from build123d import *

# Parameters (mm, degrees)
SKETCH_1_R               = 9
EXTRUDE_1_DEPTH          = 7.5
SKETCH_2_R               = 5
EXTRUDE_2_DEPTH          = 6.5
SKETCH_3_R               = 3
CUT_EXTRUDE_1_DEPTH      = 19.920887928
CUT_EXTRUDE_2_DEPTH      = 19.920887928
CUT_EXTRUDE_2_DEPTH_BACK = 19.920887928
SKETCH_4_R               = 1.5
SKETCH_5_W               = 4
SKETCH_5_H               = 1
SKETCH_6_R               = 0.75
CUT_EXTRUDE_3_DEPTH      = 10
CUT_EXTRUDE_4_DEPTH      = 19.920888002
CUT_EXTRUDE_4_DEPTH_BACK = 19.920888002
SKETCH_8_W               = 6.5
SKETCH_8_H               = 0.5


with BuildPart() as part:
    # 草图1 → 凸台-拉伸1 (new body)
    with BuildSketch(Plane.XY):
        Circle(SKETCH_1_R)
    extrude(amount=EXTRUDE_1_DEPTH)

    # 草图2 → 凸台-拉伸2 (add)
    with BuildSketch(Plane.XY.offset(7.5)):
        with Locations(Location((0, 0, 0), (0, 0, 180))):
            Circle(SKETCH_2_R)
    extrude(amount=EXTRUDE_2_DEPTH)

    # 草图3 → 切除-拉伸1 (cut, through all)
    with BuildSketch(Plane.XY.offset(14)):
        Circle(SKETCH_3_R)
    extrude(amount=-CUT_EXTRUDE_1_DEPTH, mode=Mode.SUBTRACT)

    # 草图4 → 切除-拉伸2 (cut, two sides: drawn at the far end of the back side and taken through both)
    with BuildSketch(Plane(origin=(0, 0, 0), x_dir=(1, 0, 0), z_dir=(0, 1, 0)).offset(-CUT_EXTRUDE_2_DEPTH_BACK)):
        with Locations(Location((0, -11, 0), (0, 0, 270))):
            Circle(SKETCH_4_R)
    extrude(amount=CUT_EXTRUDE_2_DEPTH + CUT_EXTRUDE_2_DEPTH_BACK, mode=Mode.SUBTRACT)

    # 草图5 → 切除-旋转1 (revolve, cut)
    with BuildSketch(Plane(origin=(0, 0, 0), x_dir=(1, 0, 0), z_dir=(0, 1, 0)), mode=Mode.PRIVATE) as cut_revolve_1_sk:
        with Locations((7, -1.5)):
            Rectangle(SKETCH_5_W, SKETCH_5_H)
        with Locations((7, -6)):
            Rectangle(SKETCH_5_W, SKETCH_5_H)
    revolve(cut_revolve_1_sk.sketch.rotate(Axis((0, 0, -0.802981009), (0, 0, 1)), 180), axis=Axis((0, 0, -0.802981009), (0, 0, 1)), mode=Mode.SUBTRACT)

    # 草图6 → 切除-拉伸3 (cut)
    with BuildSketch(Plane.XY.offset(7.5)):
        with Locations((7, 0)):
            Circle(SKETCH_6_R)
    extrude(amount=-CUT_EXTRUDE_3_DEPTH, mode=Mode.SUBTRACT)

    # 草图8 → 切除-拉伸4 (cut, two sides: drawn at the far end of the back side and taken through both)
    with BuildSketch(Plane(origin=(0, 0, 0), x_dir=(0, 0, -1), z_dir=(1, 0, 0)).offset(-CUT_EXTRUDE_4_DEPTH_BACK)):
        with Locations((-10.75, 4.75)):
            Rectangle(SKETCH_8_W, SKETCH_8_H)
    extrude(amount=CUT_EXTRUDE_4_DEPTH + CUT_EXTRUDE_4_DEPTH_BACK, mode=Mode.SUBTRACT)


solid = part.part
Model file for the job. Use its own axes, mm. A direction names the side the tool comes from. Give positions to 0.01 mm unless a question says otherwise; leave off trailing zeros. Write each loop counter-clockwise with the first axis right and the second up, starting at its lowest first coordinate (ties: lowest second). Pieces come first, ordered by that corner, then holes. Notation, with made-up numbers: (35.5, -13.75) -> (69.5, -13.75) arc R32 cw to (69.5, 21.25) -> close; hole circle Ø3 at (-9, 75.5). An arc over 180 degrees is marked (long way). Write item = value, one per line.
(1) Slice it at B-B, the plane x = 7. Give the cut face in (y, z), then the cut area to 3 significant figures.
Determined:
outline = (-5.66, 0) -> (-0.75, 0) -> (-0.75, 1) -> (-5.66, 1) -> close; (-5.66, 2) -> (-0.75, 2) -> (-0.75, 5.5) -> (-5.66, 5.5) -> close; (-5.66, 6.5) -> (-0.75, 6.5) -> (-0.75, 7.5) -> (-5.66, 7.5) -> close; (0.75, 0) -> (5.66, 0) -> (5.66, 1) -> (0.75, 1) -> close; (0.75, 2) -> (5.66, 2) -> (5.66, 5.5) -> (0.75, 5.5) -> close; (0.75, 6.5) -> (5.66, 6.5) -> (5.66, 7.5) -> (0.75, 7.5) -> close
area = 54.0 mm2
(2) Mould opens along X. For faces 4 (the face through (-1.172, 8.923, 3.726)), 5 (the face through (4, 4, 2)), 6 (the face through (2.77, -1.15, 7.1)) say: released by +X, released by -X, zero draft, split by the parting line, or undercut.
Determined:
face_4 = split by the parting line
face_5 = zero draft
face_6 = undercut
(3) Slice it at A-A, the plane y = 6.5. Give the cut face in (x, z).
Determined:
outline = (-6.22, 0) -> (6.22, 0) -> (6.22, 1) -> (-6.22, 1) -> close; (-6.22, 2) -> (6.22, 2) -> (6.22, 5.5) -> (-6.22, 5.5) -> close; (-6.22, 6.5) -> (6.22, 6.5) -> (6.22, 7.5) -> (-6.22, 7.5) -> close
(4) Probe line 1 along Z through (x, y) = (-7.25, -3.5); line 2 along Z through (x, y) = (0, 3.6); line 3 along Y through (x, z) = (0, 3). List the from-to ranges inside material, lowest first.
Determined:
line_1 = 0 to 1, 2 to 5.5, 6.5 to 7.5
line_2 = 0 to 9.5, 12.5 to 14
line_3 = -9 to -3, 3 to 9
(5) Flat gauge pins, fed straight in: P1, Ø5, axis at x = -0.5, z = 12.5, coming from the +Y side; P2, Ø10, axis at x = -4, y = 4, coming from the -Z side; P3, Ø1.5, axis at y = 5, z = 12.5, coming from the -X side; P4, Ø1, axis at y = -1.5, z = 4, coming from the +X side. Where does each tip first touch, or does it go through?
Determined:
P1 = 4.5
P2 = 0
P3 = -2.63
P4 = 8.94
(6) Slice it at D-D, the plane z = 11. Give the cut face in (x, y).
Determined:
outline = (-2.18, 4.5) arc R5 ccw to (-1.5, -4.77) -> (-1.5, -2.6) arc R3 cw to (-1.5, 2.6) -> (-1.5, 4.5) -> close; (1.5, -4.77) arc R5 ccw to (2.18, 4.5) -> (1.5, 4.5) -> (1.5, 2.6) arc R3 cw to (1.5, -2.6) -> close
(7) Slice it at C-C, the plane y = -1. Give the cut face in (x, z), then the cut area to 3 significant figures.
Determined:
outline = (-8.94, 0) -> (-2.83, 0) -> (-2.83, 14) -> (-4.9, 14) -> (-4.9, 7.5) -> (-8.94, 7.5) -> (-8.94, 6.5) -> (-4.9, 6.5) -> (-4.9, 5.5) -> (-8.94, 5.5) -> (-8.94, 2) -> (-4.9, 2) -> (-4.9, 1) -> (-8.94, 1) -> close; (2.83, 0) -> (8.94, 0) -> (8.94, 1) -> (4.9, 1) -> (4.9, 2) -> (8.94, 2) -> (8.94, 5.5) -> (4.9, 5.5) -> (4.9, 6.5) -> (8.94, 6.5) -> (8.94, 7.5) -> (4.9, 7.5) -> (4.9, 14) -> (2.83, 14) -> close
area = 102 mm2
(8) Tool access for faces 1 (the face through (0, 4.5, 9)), 2 (the face through (4, -4, 7.5)), 3 (the face through (4, 4, 6.5)): list every direction of +Z, -Z, +X, -X, +Y, -Y with a clear straight run to the whole face (end or side of a thin tool).
Determined:
face_1 = +Z, +X, -X, +Y
face_2 = +Z
face_3 = none
